Could you check a few things on this model? Use its own coordinates, in mm. Face numbers are marked on the shaded views. A direction names the side the tool comes from. Give positions to 0.01 mm unless a question says otherwise; leave off trailing zeros. Loops run counter-clockwise (first coordinate to the right, second up) from the corner with the lowest first, then second, coordinate; pieces in that order, holes last. Notation, with made-up numbers: M -31,28 L 26,28 A19 ccw 26,55 Z; hole C 69.5,60 d6. An arc over 180 degrees is marked long. Answer in a Markdown table with one row per item. Add a question column.
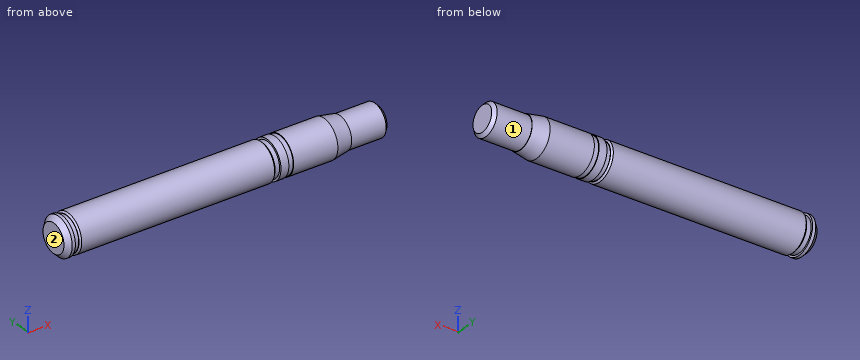
```python
from build123d import *

# Parameters (mm, degrees)
CHANFREIN1_SIZE = 1
CHANFREIN2_SIZE = 1.5
CHANFREIN3_SIZE = 0.5


with BuildPart() as part:
    # Esquisse1 → Révolution1 (revolve)
    with BuildSketch(Plane.XY, mode=Mode.PRIVATE) as r_volution1_sk:
        Polygon((-64.788489135, 0), (-64.788489135, 6), (-62.288489135, 6), (-62.288489135, 5.4), (-60.788489135, 5.4), (-60.788489135, 6), (1.211510865, 6), (1.211510865, 5.4), (2.711510865, 5.4), (2.711510865, 6), (5.211510865, 6), (5.211510865, 5.8), (6.711510865, 5.8), (6.711510865, 6), (20.711510865, 6), (25.711510865, 5.118365096), (25.711510865, 5), (37.711510865, 5), (37.711510865, 0), align=None)
    revolve(r_volution1_sk.sketch.rotate(Axis((-77.674282493, 0, 0), (1, 0, 0)), 90), axis=Axis((-77.674282493, 0, 0), (1, 0, 0)))

    # Chanfrein1
    chanfrein1_edges = [part.edges().sort_by_distance(p)[0] for p in [
        (37.711510865, 0, -5),
    ]]
    chamfer(chanfrein1_edges, length=CHANFREIN1_SIZE)

    # Chanfrein2
    chanfrein2_edges = [part.edges().sort_by_distance(p)[0] for p in [
        (-64.788489135, 0, -6),
    ]]
    chamfer(chanfrein2_edges, length=CHANFREIN2_SIZE)

    # Chanfrein3
    chanfrein3_edges = [part.edges().sort_by_distance(p)[0] for p in [
        (1.211510865, 0, -6),
        (-60.788489135, 0, -6),
    ]]
    chamfer(chanfrein3_edges, length=CHANFREIN3_SIZE)


solid = part.part
```
Item 1: Suppose I cut it at A-A (x = -16.5). List the corners of the cut face in (y, z) for me.
Item 2: I need wall thicknesses on L1, parallel to Z at x = -0.5, y = 1.5; L2, parallel to Z at x = 8.5, y = -0.25. Which ranges of each line are inside material? Lowest first, please.
Item 3: For the marked faces 1 and 2, which set-ups out of +Z, -Z, +X, -X, +Y, -Y let a thin tool reach every point of the face, with its end or its side?
Item 4: For P1, Ø4, axis at x = 11, y = -4, coming from the -Z side; P2, Ø3, axis at x = -18, z = 1.5, coming from the +Y side; P3, Ø1, axis at x = 2, z = 4, coming from the -Y side; P4, Ø1, axis at x = 27, y = 2.5, coming from the -Z side, each with a flat end and sliding along its axis, tell me the tip position at first contact or that it passes through.
Values found:
| question | item | result |
|---|---|---|
| 1 | outline | C 0,0 d12 |
| 2 | L1 | -5.81 to 5.81 |
| 2 | L2 | -5.99 to 5.99 |
| 3 | face 1 | +X |
| 3 | face 2 | +Z, -Z, -X, +Y, -Y |
| 4 | P1 | z = -5.66 |
| 4 | P2 | y = 6 |
| 4 | P3 | y = -4.11 |
| 4 | P4 | z = -4.58 |
